Autodesk Inventor part; units mm, degrees
ref_plane "YZ Plane" through (0, 0, 0) normal (1, 0, 0) x (0, 1, 0)
ref_plane "XZ Plane" through (0, 0, 0) normal (0, 1, 0) x (-1, 0, 0)
ref_plane "XY Plane" through (0, 0, 0) normal (0, 0, 1) x (1, 0, 0)
sketch "Sketch1" plane through (0, 0, 0) normal (0, 0, 1) x (1, 0, 0)
  line L0 (-180.975, -30.3906) -> (180.975, -30.3906)
  line L1 (180.975, -30.3906) -> (180.975, -106.5906)
  line L2 (180.975, -106.5906) -> (-180.975, -106.5906)
  line L3 (-180.975, -106.5906) -> (-180.975, -30.3906)
  line L4 (0, 21.3181) -> (0, -127.9087)
  point P0 (0, 0)
  dimension "d0" = 361.95
  dimension "d1" = 76.2
  dimension "d4" = 180.975
extrude "Extrusion1" add sketch "Sketch1" along normal blind 19.05
sketch "Sketch2" plane through (0, 0, 19.05) normal (0, 0, 1) x (1, 0, 0)
  line L0 (0, 21.3181) -> (0, -127.9087)
  line L1 (180.975, -30.3906) -> (-180.975, -30.3906)
  line L2 (-60.325, -30.3906) -> (60.325, -30.3906)
  line L3 (60.325, -30.3906) -> (60.325, -68.4906)
  line L4 (60.325, -68.4906) -> (-60.325, -68.4906)
  line L5 (-60.325, -68.4906) -> (-60.325, -30.3906)
  point P0 (0, 0)
  dimension "d5" = 120.65
  dimension "d6" = 60.325
  dimension "d7" = 38.1
extrude "Extrusion2" cut sketch "Sketch2" against normal blind 19.05
fillet "Fillet1" radius 19.05 4 edges at (-60.325, -30.3906, 9.525) (60.325, -30.3906, 9.525) (60.325, -68.4906, 9.525) (-60.325, -68.4906, 9.525)
equation "\"d4\" = 0.5 * d0"
equation "\"d5\" = 0.333333 * d0"
equation "\"d6\" = 0.5 * d5"
properties part number "Drawer ends" material "Wood (Cherry)"
Check sheet for the modelled part. Datum: model origin and axes. Units: mm. A direction names the side the tool comes from. Round coordinates to 2 decimals unless told otherwise and drop trailing zeros. Loops run counter-clockwise (first coordinate to the right, second up) from the corner with the lowest first, then second, coordinate; pieces in that order, holes last. Notation, with made-up numbers: (34.5, 66) -> (47.5, 66) arc R11 cw to (47.5, 82) -> close; hole circle Ø2 at (26, 32). An arc over 180 degrees is marked (long way). Put each result on its own line as item: value. Start each with the question number.
1. Section check C-C (y = -63). Enter the section's corners in (x, z) (3 decimals).
2. Draft check along X on faces 1 (the face through (-66.053, -35.823, 9.392)), 2 (the face through (65.757, -36.119, 9.392)), 3 (the face through (180.975, -68, 9)), 4 (the face through (-3, -76, 19.05)). Enter one of: +X half, -X half, draft (parallel to the pull), parting line (faces both ways), or undercut.
3. Section check D-D (x = -15.5). Enter the section's corners in (y, z).
4. Access from +Z, -Z, +X, -X, +Y, -Y to the whole of each face (thin tool, end or side, straight path). Record for faces 5 (the face through (1, -68.491, 10)), 6 (the face through (129, -30.391, 9)).
5. Gauge pin test, flat end, axial feed: pin 1 (9.5 mm diameter, centred on x = 12.5, z = 7, fed in from +Y). Record the tip position at first contact, or that the pin passes through.
6. Scan lines: probe 1 along Y at (x, z) = (19, 9.5); probe 2 along X at (y, z) = (-65.5, 1.25) (3 decimals); probe 3 along X at (y, z) = (-37.5, 2) (3 decimals). Record each from-to range of solid material in increasing order.
7. Section check A-A (y = -40). Enter the section's corners in (x, z) (3 decimals).
Findings:
1. outline: (-180.975, 0) -> (-54.656, 0) -> (-54.656, 19.05) -> (-180.975, 19.05) -> close; (54.656, 0) -> (180.975, 0) -> (180.975, 19.05) -> (54.656, 19.05) -> close
2. face 1: undercut
2. face 2: undercut
2. face 3: +X half
2. face 4: draft
3. outline: (-106.59, 0) -> (-68.49, 0) -> (-68.49, 19.05) -> (-106.59, 19.05) -> close
4. face 5: +Z, -Z, +Y
4. face 6: +Z, -Z, +X, -X, +Y
5. pin 1: stops at y = -68.49
6. probe 1: y = -106.59 to -68.49
6. probe 2: x = -180.975 to -51.522, 51.522 to 180.975
6. probe 3: x = -180.975 to -64.531, 64.531 to 180.975
7. outline: (-180.975, 0) -> (-62.829, 0) -> (-62.829, 19.05) -> (-180.975, 19.05) -> close; (62.829, 0) -> (180.975, 0) -> (180.975, 19.05) -> (62.829, 19.05) -> close
